```python
from build123d import *

# Parameters (mm, degrees)
SKETCH1_W           = 38
SKETCH1_H           = 24.5
SKETCH1_R           = 8.3
BOSS_EXTRUDE1_DEPTH = 8.5
FILLET1_R           = 15
FILLET2_R           = 1
CHAMFER1_SIZE       = 1


with BuildPart() as part:
    # Sketch1 → Boss-Extrude1 (new body)
    with BuildSketch(Plane(origin=(0, 0, 0), x_dir=(1, 0, 0), z_dir=(0, 1, 0))):
        Rectangle(SKETCH1_W, SKETCH1_H)
        with Locations(Location((0, 0, 0), (0, 0, 270))):
            Circle(SKETCH1_R, mode=Mode.SUBTRACT)
    extrude(amount=BOSS_EXTRUDE1_DEPTH)

    # Fillet1
    fillet1_edges = [part.edges().sort_by_distance(p)[0] for p in [
        (19, 4.25, 12.25),
        (-19, 4.25, 12.25),
    ]]
    fillet(fillet1_edges, radius=FILLET1_R)

    # Fillet2
    fillet2_edges = [part.edges().sort_by_distance(p)[0] for p in [
        (-19, 4.25, -12.25),
        (19, 4.25, -12.25),
    ]]
    fillet(fillet2_edges, radius=FILLET2_R)

    # Chamfer1
    chamfer1_edges = [part.edges().sort_by_distance(p)[0] for p in [
        (0, 8.5, -8.3),
    ]]
    chamfer(chamfer1_edges, length=CHAMFER1_SIZE)


solid = part.part
```
Work out the finished part from the listing and answer in its coordinate system (mm). Give positions to 0.01 mm unless a question says otherwise; leave off trailing zeros. Order: outer loops, then holes, each group sorted by start corner. A loop starts at its lowest first (then second) coordinate and runs counter-clockwise, first axis right, second up.
1. Section A-A, the plane x = 0 is taken. Determine the outline of the cut face in (y, z), and give its area (4 significant figures).
Result sheet:
outline: (0, -12.25) - (8.5, -12.25) - (8.5, -9.3) - (7.5, -8.3) - (0, -8.3) - close; (0, 8.3) - (7.5, 8.3) - (8.5, 9.3) - (8.5, 12.25) - (0, 12.25) - close
area: 66.15 mm2
2. Section B-B, the plane y = 4.75 is taken. Determine the outline of the cut face in (x, z).
Result sheet:
outline: (-19, -11.25) arc R1 ccw to (-18, -12.25) - (18, -12.25) arc R1 ccw to (19, -11.25) - (19, -2.75) arc R15 ccw to (4, 12.25) - (-4, 12.25) arc R15 ccw to (-19, -2.75) - close; hole circle Ø16.6 at (0, 0)
3. The mould has two halves that part along Z. Classify faces 1 (the flat face through (4, 0, -8)), 2 (the cylindrical face through (-5.05, 3.698, -6.587)), 3 (the flat face through (0, 4, 12.25)): released by +Z, released by -Z, zero draft, split by the parting line, or undercut.
Result sheet:
face 1: zero draft
face 2: undercut
face 3: released by +Z
4. Straight lines are drawn through the part: L1, parallel to X at y = 2.25, z = 0; L2, parallel to Z at x = -7.5, y = 2.5; L3, parallel to X at y = 4.25, z = 3.5. For each, find the intervals that lie inside material, in ascending order.
Result sheet:
L1: x = -18.75 to -8.3, 8.3 to 18.75
L2: z = -12.25 to -3.56, 3.56 to 11.84
L3: x = -17.64 to -7.53, 7.53 to 17.64
5. Section C-C, the plane z = 0 is taken. Determine the outline of the cut face in (x, y), and give its area (3 significant figures).
Result sheet:
outline: (-18.75, 0) - (-8.3, 0) - (-8.3, 7.5) - (-9.3, 8.5) - (-18.75, 8.5) - close; (8.3, 0) - (18.75, 0) - (18.75, 8.5) - (9.3, 8.5) - (8.3, 7.5) - close
area: 177 mm2
6. Each of these flat-tipped pins is pushed along its axis until it touches: P1, Ø10, axis at x = -1, z = 3, coming from the -Y side; P2, Ø1, axis at y = 4.5, z = -1.5, coming from the -X side. Where does it stop, or does it pass through?
Result sheet:
P1: passes through
P2: stops at x = -18.98
7. Section D-D, the plane x = -11 is taken. Determine the outline of the cut face in (y, z), and give its area (3 significant figures).
Result sheet:
outline: (0, -12.25) - (8.5, -12.25) - (8.5, 10.52) - (0, 10.52) - close
area: 194 mm2
